Print and shaded views of the part. All mm, measured from the part's lowest x, y and z. A direction names the side the tool comes from. Coordinates: 2 decimals unless noted, no trailing zeros. Loops run counter-clockwise (first coordinate to the right, second up) from the corner with the lowest first, then second, coordinate; pieces in that order, holes last.
1) Two-plate mould, pull along Z, no slides. Class the marked faces 3, 4, 5 and 6: +Z half, -Z half, draft (parallel to the pull), parting line (faces both ways), or undercut.
2) Saw through at A-A, the plane z = 19.5. Write the cut outline in (x, y) (3 decimals).
3) Which spindle directions (+Z, -Z, +X, -X, +Y, -Y) get a long thin tool onto all of the face, cutting with end or side? Do the marked faces 1 and 2. Say none if no direction does.
4) Wall check: line 1 along Z through (x, y) = (43, 32) (3 decimals); line 2 along X through (y, z) = (18.5, 32.5) (3 decimals); line 3 along X through (y, z) = (43, 7). Give the ranges that are in metal, low to high.
5) Saw through at C-C, the plane y = 40.5. Write the cut outline in (x, z) (3 decimals).
6) Saw through at B-B, the plane x = 47.5. Write the cut outline in (y, z) (3 decimals).
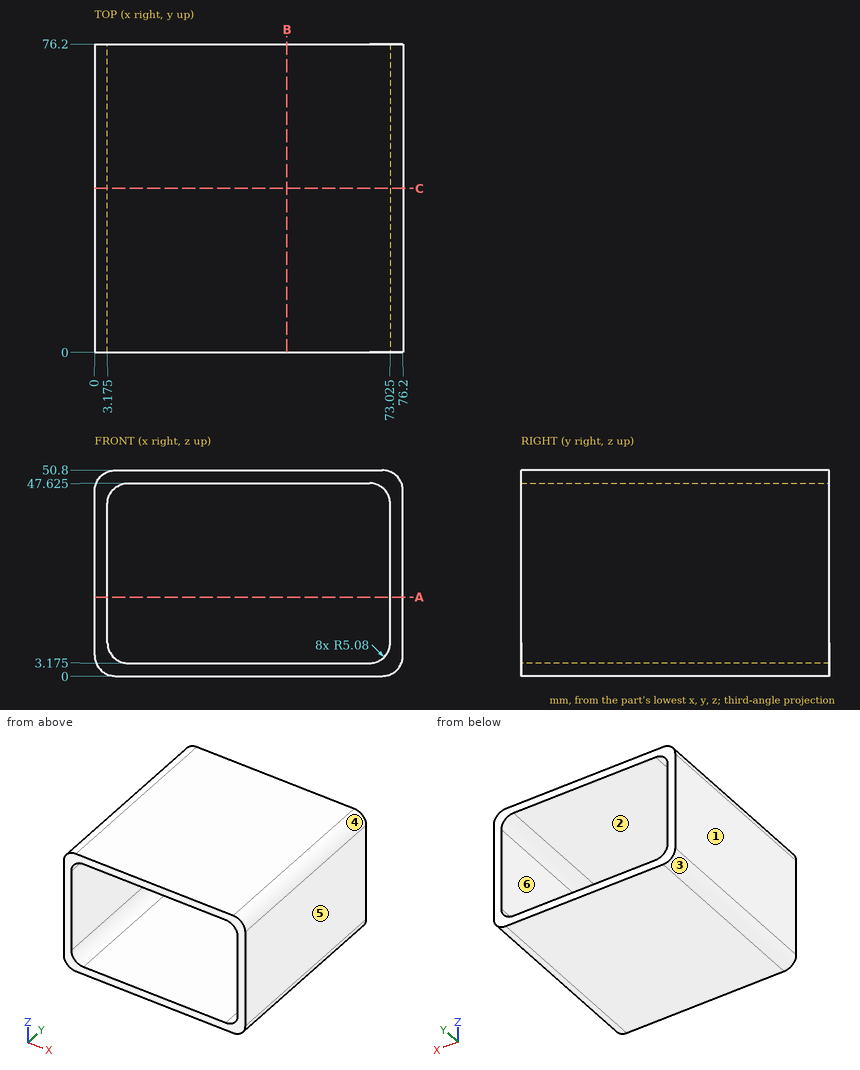
Data:
1. face 3: -Z half
1. face 4: +Z half
1. face 5: draft
1. face 6: undercut
2. outline: (0, 0) - (3.175, 0) - (3.175, 76.2) - (0, 76.2) - close; (73.025, 0) - (76.2, 0) - (76.2, 76.2) - (73.025, 76.2) - close
3. face 1: +Z, -Z, -X, +Y, -Y
3. face 2: +Y, -Y
4. line 1: z = 0 to 3.175, 47.625 to 50.8
4. line 2: x = 0 to 3.175, 73.025 to 76.2
4. line 3: x = 0 to 3.33, 72.87 to 76.2
5. outline: (0, 5.08) arc R5.08 ccw to (5.08, 0) - (71.12, 0) arc R5.08 ccw to (76.2, 5.08) - (76.2, 45.72) arc R5.08 ccw to (71.12, 50.8) - (5.08, 50.8) arc R5.08 ccw to (0, 45.72) - close; hole (3.175, 8.255) arc R5.08 ccw to (8.255, 3.175) - (67.945, 3.175) arc R5.08 ccw to (73.025, 8.255) - (73.025, 42.545) arc R5.08 ccw to (67.945, 47.625) - (8.255, 47.625) arc R5.08 ccw to (3.175, 42.545) - close
6. outline: (0, 0) - (76.2, 0) - (76.2, 3.175) - (0, 3.175) - close; (0, 47.625) - (76.2, 47.625) - (76.2, 50.8) - (0, 50.8) - close
